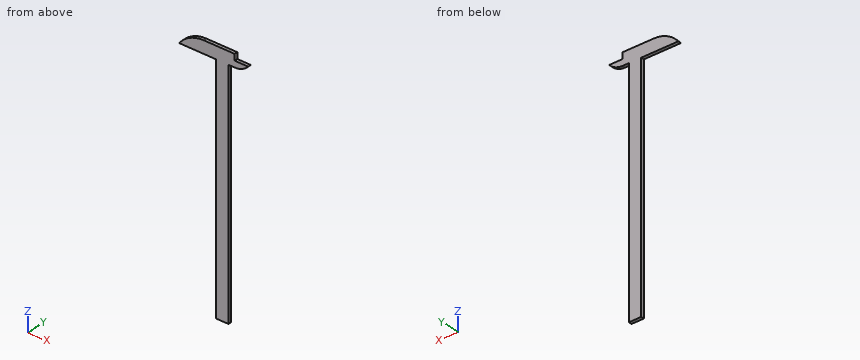
from build123d import *

# Parameters (mm, degrees)
F0_W     = 12.7
F0_H     = 241.3
F0_H_2   = 12.7
F1_DEPTH = 1.651


with BuildPart() as f1:
    # F0 (on Front) → F1 (new body, symmetric)
    with BuildSketch(Plane.XZ):
        Rectangle(F0_W, F0_H)
        Polygon((6.35, 133.35), (6.35, 120.65), (12.7, 120.65), (12.7, 127), (12.7, 133.35), align=None)
        with Locations((0, 127)):
            Rectangle(F0_W, F0_H_2)
        with BuildLine():
            Line((-44.45, 120.65), (-6.35, 120.65))
            Line((-6.35, 120.65), (-6.35, 133.35))
            Line((-6.35, 133.35), (-19.05, 133.35))
            ThreePointArc((-19.05, 133.35), (-33.249032, 129.998063), (-44.45, 120.65))
        make_face()
        with BuildLine():
            Line((12.7, 127), (12.7, 120.65))
            ThreePointArc((12.7, 120.65), (20.372734, 122.311985), (26.67, 127))
            Line((26.67, 127), (12.7, 127))
        make_face()
    extrude(amount=F1_DEPTH, both=True)


solid = f1.part
Input: part model. Units: mm. Frame: model coordinates. Give positions to 0.01 mm unless a question says otherwise; leave off trailing zeros. Write each loop counter-clockwise with the first axis right and the second up, starting at its lowest first coordinate (ties: lowest second). Pieces come first, ordered by that corner, then holes.
Q1. First-contact query: P1, Ø1.7, axis at x = 22, y = 0.5, coming from the +Z side; P2, Ø1, axis at y = 0, z = 129, coming from the +X side; P3, Ø1, axis at y = 0, z = -31.5, coming from the +X side. Flat tips, straight axial feed; report the tip coordinate or a pass-through.
Q2. Section B-B, the plane z = 86.5. Output: boundary loops of the cut face in (x, y).
Q3. Material intervals for probe 1 along X at (y, z) = (-0.2, 82.5); probe 2 along Z at (x, y) = (-12.5, -1.2); probe 3 along Z at (x, y) = (-24, 0.4), sorted ascending.
Q4. Section C-C, the plane x = -25. Output: boundary loops of the cut face in (y, z).
Q5. Section A-A, the plane y = -1. Output: boundary loops of the cut face in (x, z).
Filled in:
1. P1: stops at z = 127
1. P2: stops at x = 12.7
1. P3: stops at x = 6.35
2. outline: (-6.35, -1.65) - (6.35, -1.65) - (6.35, 1.65) - (-6.35, 1.65) - close
3. probe 1: x = -6.35 to 6.35
3. probe 2: z = 120.65 to 133.35
3. probe 3: z = 120.65 to 132.96
4. outline: (-1.65, 120.65) - (1.65, 120.65) - (1.65, 132.79) - (-1.65, 132.79) - close
5. outline: (-44.45, 120.65) - (-6.35, 120.65) - (-6.35, -120.65) - (6.35, -120.65) - (6.35, 120.65) - (12.7, 120.65) arc R18.54 ccw to (26.67, 127) - (12.7, 127) - (12.7, 133.35) - (-19.05, 133.35) arc R31.75 ccw to start
